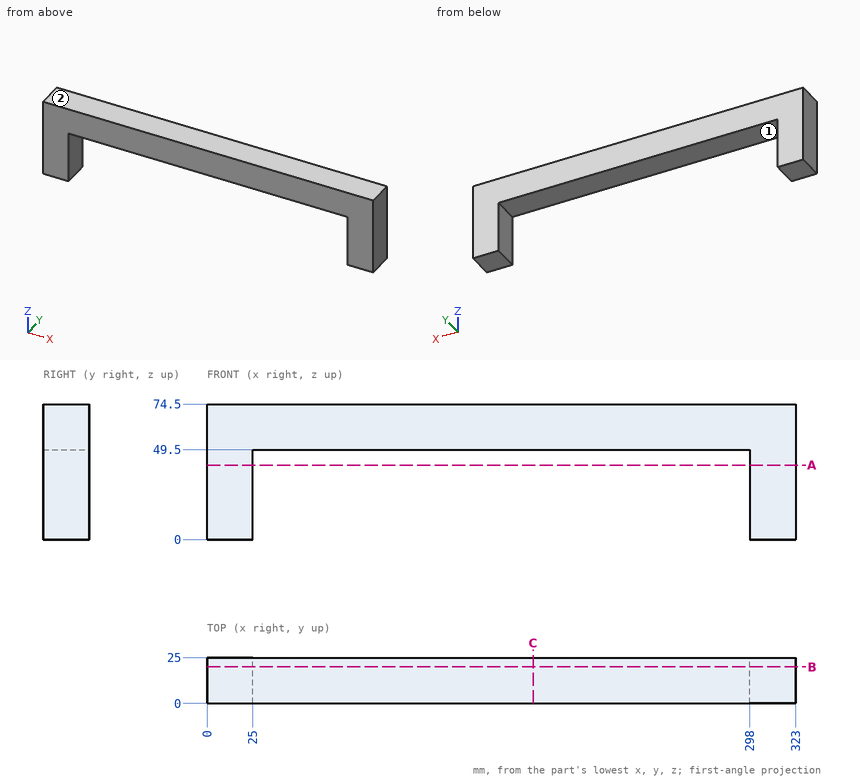
Drawing for the job (mm, zero at the part's lowest x, y, z). Give positions to 0.01 mm unless a question says otherwise; leave off trailing zeros. Order: outer loops, then holes, each group sorted by start corner. A loop starts at its lowest first (then second) coordinate and runs counter-clockwise, first axis right, second up. Notation, with made-up numbers: (84, 34) - (142, 34) arc R15 ccw to (142, 41) - close; hole circle Ø1 at (-12, 77.25). An arc over 180 degrees is marked (long way). Use one line per item in the form item = value.
Item 1: Slice it at A-A on z = 41. Give the cut face in (x, y).
Solution:
outline = (0, 0) - (25, 0) - (25, 25) - (0, 25) - close; (298, 0) - (323, 0) - (323, 25) - (298, 25) - close
Item 2: Pin check, flat tip, straight feed: pin 1 Ø6 at (x, y) = (263, 20) entering from -Z. Stop position of the tip, or through.
Solution:
pin_1 = 49.5
Item 3: Probe probe 1 along X at (y, z) = (3, 24.5); probe 2 along Z at (x, y) = (275.5, 7.75). List the from-to ranges inside material, lowest first. Write a range as from..to.
Solution:
probe_1 = 0..25, 298..323
probe_2 = 49.5..74.5
Item 4: Two-plate mould, pull along X, no slides. Class the marked faces 1 and 2: released by +X, released by -X, zero draft, split by the parting line, or undercut.
Solution:
face_1 = undercut
face_2 = zero draft
Item 5: Slice it at C-C on x = 179. Give the cut face in (y, z), and give its area (3 significant figures).
Solution:
outline = (0, 49.5) - (25, 49.5) - (25, 74.5) - (0, 74.5) - close
area = 625 mm2
Item 6: Slice it at B-B on y = 20. Give the cut face in (x, z), and give its area (4 significant figures).
Solution:
outline = (0, 0) - (25, 0) - (25, 49.5) - (298, 49.5) - (298, 0) - (323, 0) - (323, 74.5) - (0, 74.5) - close
area = 10,550 mm2
